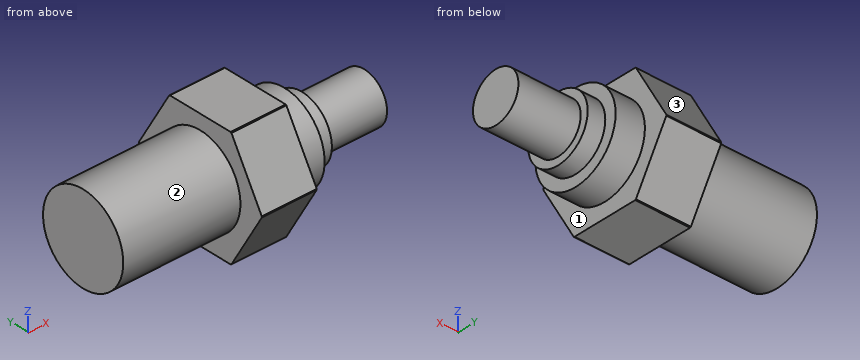
```python
from build123d import *

# Parameters (mm, degrees)
F3_START = 13.9
F3_DEPTH = 38.9


with BuildPart() as f1:
    # F0 (on Top) → F1 (revolve)
    with BuildSketch(Plane.XY):
        Polygon((-9.9245372606, 3), (-9.9245372606, 0), (9.2754627394, 0), (9.2754627394, 1.7), (5.0254627394, 1.7), (5.0254627394, 2.225), (3.8254627394, 2.225), (3.8254627394, 3), (1.8254627394, 3), (1.8254627394, 4.6), (-1.9245372606, 4.6), (-1.9245372606, 3), align=None)
    revolve(axis=Axis((-0.3245372606, 0, 0), (1, 0, 0)))

    # F2 (on face) → F3 (intersect)
    with BuildSketch(Plane(origin=(-1.9245372606, 0, 0), x_dir=(0, -1, 0), z_dir=(-1, 0, 0)).offset(F3_START)):
        Polygon((2.3094010768, 4), (-2.3094010768, 4), (-4.6188021535, 0), (-2.3094010768, -4), (2.3094010768, -4), (4.6188021535, 0), align=None)
    extrude(amount=-F3_DEPTH, mode=Mode.INTERSECT)


solid = f1.part
```
The listing builds one solid part. Answer for the finished solid, in the listing's coordinates (mm). Face numbers are marked on the shaded views. A direction names the side the tool comes from. Give positions to 0.01 mm unless a question says otherwise; leave off trailing zeros. Order: outer loops, then holes, each group sorted by start corner. A loop starts at its lowest first (then second) coordinate and runs counter-clockwise, first axis right, second up. Notation, with made-up numbers: (72.5, 84.5) -> (96.5, 84.5) arc R21 cw to (96.5, 118.5) -> close; hole circle Ø3 at (3, 55). An arc over 180 degrees is marked (long way). Answer as CSV lines item,"result". Start each with the question number.
Q1. Given pin 1 (1 mm diameter, centred on x = -5.5, y = -1, fed in from +Z); pin 2 (1.5 mm diameter, centred on x = -3, y = 2.5, fed in from -Z); pin 3 (4 mm diameter, centred on x = -6.5, y = 3.5, fed in from +Z), each flat-ended and moving along its own axis, determine where each tip first touches the part or whether it passes through.
Q2. A cutting plane is placed at D-D (z = 2). Determine the outline of the cut face in (x, y) (3 decimals), then the cut area to 3 significant figures.
Q3. A cutting plane is placed at A-A (y = 0). Determine the outline of the cut face in (x, z) (3 decimals).
Q4. A cutting plane is placed at C-C (z = -0.5). Determine the outline of the cut face in (x, y), then the cut area to 3 significant figures.
Q5. Which of the six approach directions +Z, -Z, +X, -X, +Y, -Y give full straight-line access (tool end or side, diameter ignored) to the marked faces 1, 2 and 3?
Q6. Find the intervals of material crossed by L1, parallel to X at y = -2.5, z = 2.5; L2, parallel to X at y = 0.75, z = 2.25; L3, parallel to Z at x = -3.25, y = -1, in increasing order.
Q7. A cutting plane is placed at B-B (x = -0.75). Determine the outline of the cut face in (y, z).
Results found:
1,pin 1,"z = 2.96"
1,pin 2,"z = -2.44"
1,pin 3,"z = 2.6"
2,outline,"(-9.925, -2.236) -> (-1.925, -2.236) -> (-1.925, -3.464) -> (1.825, -3.464) -> (1.825, -2.236) -> (3.825, -2.236) -> (3.825, -0.975) -> (5.025, -0.975) -> (5.025, 0.975) -> (3.825, 0.975) -> (3.825, 2.236) -> (1.825, 2.236) -> (1.825, 3.464) -> (-1.925, 3.464) -> (-1.925, 2.236) -> (-9.925, 2.236) -> close"
2,area,"73.0 mm2"
3,outline,"(-9.925, -3) -> (-1.925, -3) -> (-1.925, -4) -> (1.825, -4) -> (1.825, -3) -> (3.825, -3) -> (3.825, -2.225) -> (5.025, -2.225) -> (5.025, -1.7) -> (9.275, -1.7) -> (9.275, 1.7) -> (5.025, 1.7) -> (5.025, 2.225) -> (3.825, 2.225) -> (3.825, 3) -> (1.825, 3) -> (1.825, 4) -> (-1.925, 4) -> (-1.925, 3) -> (-9.925, 3) -> close"
4,outline,"(-9.92, -2.96) -> (-1.92, -2.96) -> (-1.92, -4.33) -> (1.83, -4.33) -> (1.83, -2.96) -> (3.83, -2.96) -> (3.83, -2.17) -> (5.03, -2.17) -> (5.03, -1.62) -> (9.28, -1.62) -> (9.28, 1.62) -> (5.03, 1.62) -> (5.03, 2.17) -> (3.83, 2.17) -> (3.83, 2.96) -> (1.83, 2.96) -> (1.83, 4.33) -> (-1.92, 4.33) -> (-1.92, 2.96) -> (-9.92, 2.96) -> close"
4,area,"111 mm2"
5,face 1,"+X"
5,face 2,"-X"
5,face 3,"+Z, +X, -X, +Y"
6,L1,"-1.92 to 1.83"
6,L2,"-9.92 to 3.83"
6,L3,"-2.83 to 2.83"
7,outline,"(-4.6, -0.03) -> (-2.33, -3.97) arc R4.6 ccw to (-2.27, -4) -> (2.27, -4) arc R4.6 ccw to (2.33, -3.97) -> (4.6, -0.03) arc R4.6 ccw to (4.6, 0.03) -> (2.33, 3.97) arc R4.6 ccw to (2.27, 4) -> (-2.27, 4) arc R4.6 ccw to (-2.33, 3.97) -> (-4.6, 0.03) arc R4.6 ccw to start"
